Geometry check sheet. Reference: drawing and pictorial views, mm from the part's lowest x, y, z. A direction names the side the tool comes from. Round coordinates to 2 decimals unless told otherwise and drop trailing zeros. Order: outer loops, then holes, each group sorted by start corner. A loop starts at its lowest first (then second) coordinate and runs counter-clockwise, first axis right, second up.
Q1. Scan lines: probe 1 along Z at (x, y) = (9, 7); probe 2 along X at (y, z) = (7.75, 5); probe 3 along Y at (x, z) = (11.75, 6.5). Record each from-to range of solid material in increasing order.
Q2. Cross-section at A-A on y = 9.75. Record the cut outline in (x, z).
Q3. Cross-section at C-C on x = 9.25. Record the cut outline in (y, z).
Q4. Mould release check, pull along X, two halves, no side actions. Record for the marked faces 3, 4 and 5: +X half, -X half, draft (parallel to the pull), parting line (faces both ways), or undercut.
Q5. Set-up check for the marked faces 1 and 2: record each of +Z, -Z, +X, -X, +Y, -Y from which the full face is reachable in a straight line by a thin tool's end or side.
Q6. Depth check by flat-ended pin: P1, Ø6, axis at x = 19.5, y = 4, coming from the -Z side; P2, Ø1, axis at x = 8.5, z = 2, coming from the +Y side; P3, Ø1.8, axis at x = 17, y = 7, coming from the -Z side. Enter the tip coordinate at first touch or a pass-through.
Q7. Cross-section at D-D on x = 18. Record the cut outline in (y, z), then the cut area to 3 significant figures.
Q8. Cross-section at B-B on z = 5. Record the cut outline in (x, y), then the cut area to 3 significant figures.
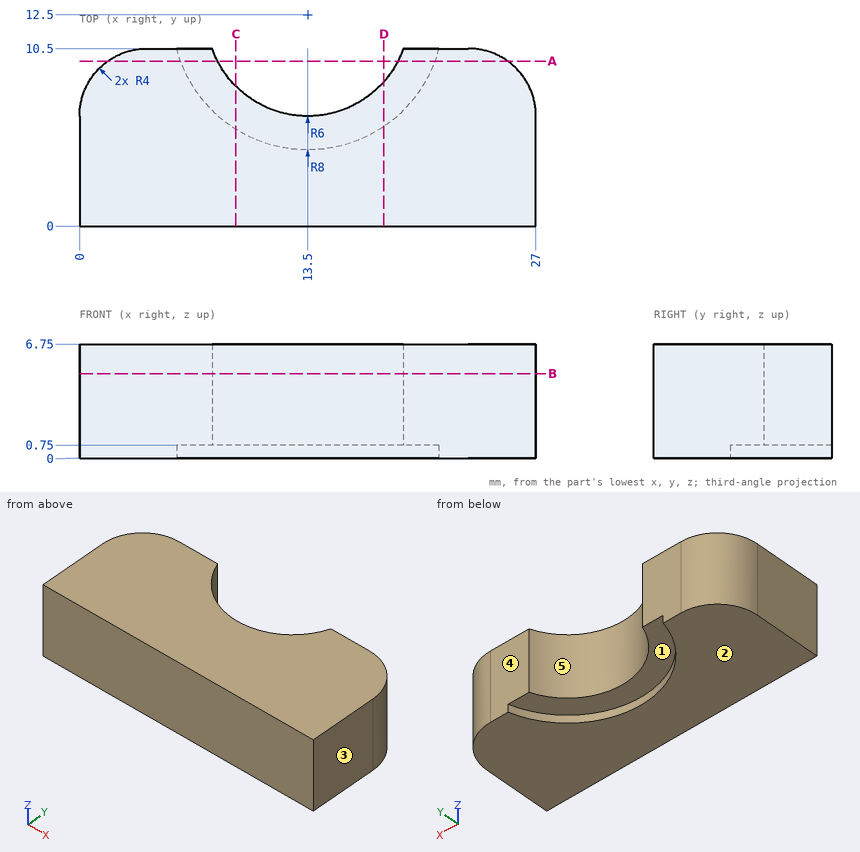
Results found:
1. probe 1: z = 0.75 to 6.75
1. probe 2: x = 0.2 to 9.83, 17.17 to 26.8
1. probe 3: y = 0 to 6.76
2. outline: (1.67, 0) - (5.99, 0) - (5.99, 0.75) - (8.17, 0.75) - (8.17, 6.75) - (1.67, 6.75) - close; (18.83, 0.75) - (21.01, 0.75) - (21.01, 0) - (25.33, 0) - (25.33, 6.75) - (18.83, 6.75) - close
3. outline: (0, 0) - (5.72, 0) - (5.72, 0.75) - (8.26, 0.75) - (8.26, 6.75) - (0, 6.75) - close
4. face 3: +X half
4. face 4: draft
4. face 5: undercut
5. face 1: -Z, +Y
5. face 2: -Z, +X, -X, +Y, -Y
6. P1: stops at z = 0
6. P2: stops at y = 10.1
6. P3: stops at z = 0.75
7. outline: (0, 0) - (5.89, 0) - (5.89, 0.75) - (8.53, 0.75) - (8.53, 6.75) - (0, 6.75) - close
7. area: 55.6 mm2
8. outline: (0, 0) - (27, 0) - (27, 6.5) arc R4 ccw to (23, 10.5) - (19.16, 10.5) arc R6 cw to (7.84, 10.5) - (4, 10.5) arc R4 ccw to (0, 6.5) - close
8. area: 244 mm2
